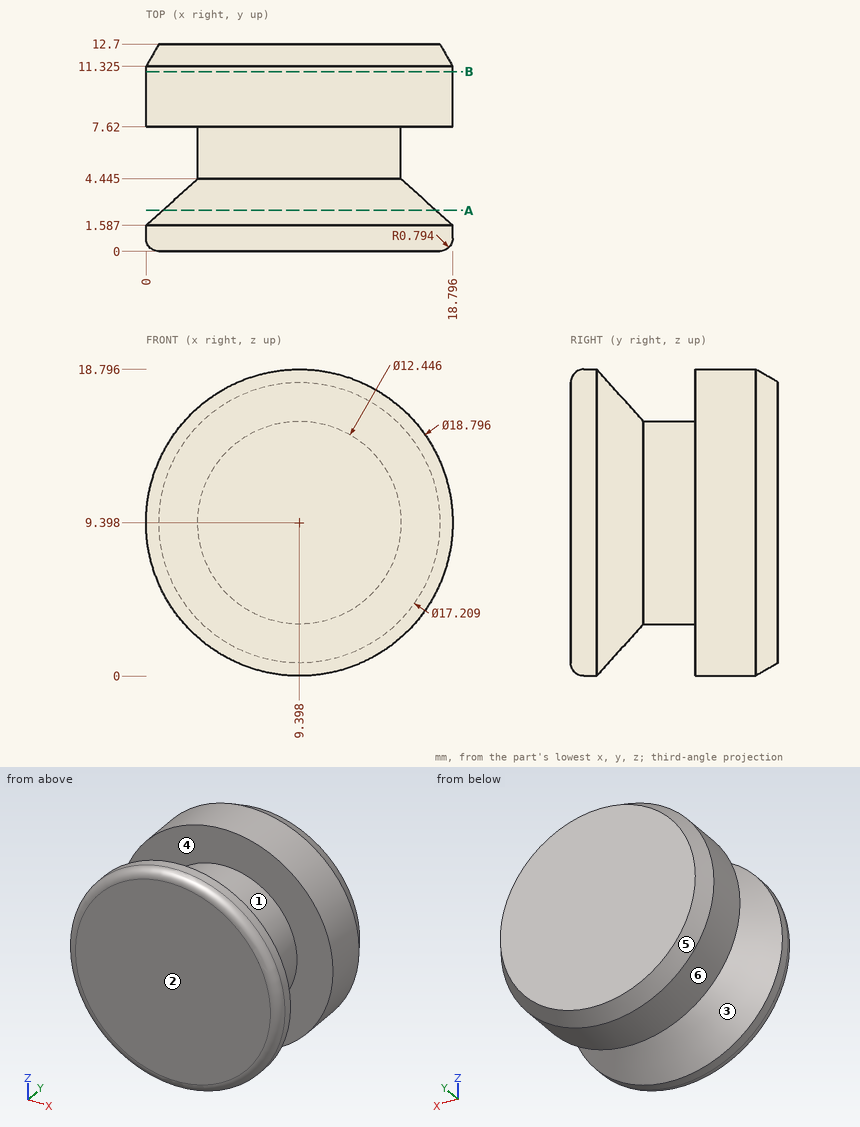
Could you check a few things on this drawing? It's one solid part, dimensions in mm from its lowest x, y, z. A direction names the side the tool comes from. Give positions to 0.01 mm unless a question says otherwise; leave off trailing zeros. Order: outer loops, then holes, each group sorted by start corner. A loop starts at its lowest first (then second) coordinate and runs counter-clockwise, first axis right, second up.
1. Which directions (+Z, -Z, +X, -X, +Y, -Y) give clear straight access to the entire face, cutting with the end or side of a thin tool? Please do the marked faces 1 and 2.
Answers below:
face 1: none
face 2: +Z, -Z, +X, -X, -Y
2. For pin 1 (3 mm diameter, centred on y = 5.5, z = 3, fed in from +X) (1 decimal); pin 2 (1.5 mm diameter, centred on y = 2.5, z = 4, fed in from +X) (1 decimal); pin 3 (4 mm diameter, centred on x = 11.5, y = 5, fed in from +Z) (1 decimal), each with a flat end and sliding along its axis, tell me the tip position at first contact or that it passes through.
Answers below:
pin 1: stops at x = 13.2
pin 2: stops at x = 17
pin 3: stops at z = 17
3. Thinking about a two-plate mould opening in Y: for the marked faces 3, 4, 5 and 6, which applies, +Y half, -Y half, draft (parallel to the pull), parting line (faces both ways), or undercut?
Answers below:
face 3: undercut
face 4: undercut
face 5: +Y half
face 6: draft
4. Suppose I cut it at B-B (y = 11). Write out the boundary of the cut face in (x, z) (1 decimal).
Answers below:
outline: circle Ø18.8 at (9.4, 9.4)
5. Suppose I cut it at A-A (y = 2.5). Write out the boundary of the cut face in (x, z) (1 decimal).
Answers below:
outline: circle Ø16.8 at (9.4, 9.4)
6. I need wall thicknesses on L1, parallel to Y at x = 16, z = 6.25 (1 decimal); L2, parallel to Y at x = 16.75, z = 11.5 (1 decimal); L3, parallel to X at y = 5.75, z = 9.25. Which ranges of each line are inside material? Lowest first, please.
Answers below:
L1: y = 0 to 3.5, 7.6 to 12.7
L2: y = 0 to 3.2, 7.6 to 12.7
L3: x = 3.18 to 15.62
